from build123d import *

# Parameters (mm, degrees)
F1_DEPTH = 80
F2_R     = 2.25
F3_DEPTH = 3
F4_R     = 1.49999


# Not quite as in the source:
# - a fillet or chamfer is up to 0.001 mm smaller than in the source, because OpenCascade refuses the exact size
# - a feature names something its author has since deleted; it is built from what else it names


with BuildPart() as f1:
    # F0 (on Top) → F1 (new body)
    with BuildSketch(Plane.XY):
        with BuildLine():
            Line((45, 3), (3, 3))
            Line((3, 3), (3, 6))
            ThreePointArc((3, 6), (29.6273152762, 21.5830013932), (60, 27))
            Line((60, 27), (60, 30))
            ThreePointArc((60, 30), (27.9372056463, 24.1546059211), (0, 7.3705672421))
            Line((0, 7.3705672421), (0, 0))
            Line((0, 0), (45, 0))
            Line((45, 0), (45, 3))
        make_face()
    extrude(amount=F1_DEPTH)

    # F2 (on face) → F3 (cut, through all)
    with BuildSketch(Plane.XZ):
        with Locations((30, 72)):
            Circle(F2_R)
        with Locations((30, 8)):
            Circle(F2_R)
    extrude(amount=-F3_DEPTH, mode=Mode.SUBTRACT)

    # F4 (radius 1.5 in the source; OpenCascade refuses exactly that, so slightly less here)
    f4_edges = [f1.edges().sort_by_distance(p)[0] for p in [
        (45, 0, 40),
        (45, 3, 40),
        (0, 0, 40),
        (0, 7.370567, 40),
        (60, 30, 40),
        (60, 27, 40),
        (3, 3, 40),
        (3, 6, 40),
    ]]
    fillet(f4_edges, radius=F4_R)


solid = f1.part
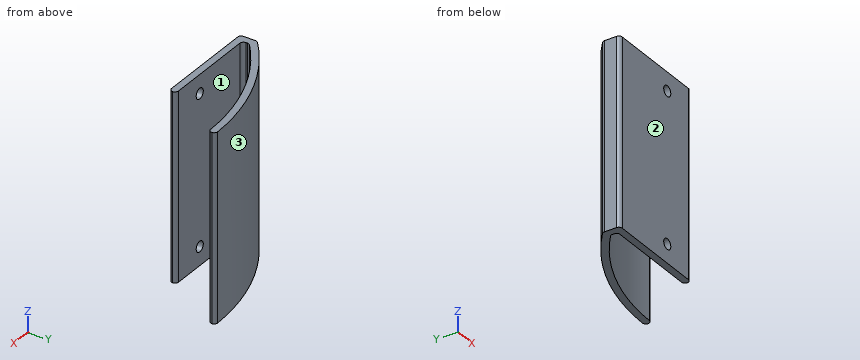
CAD build for the part. Positions are in the model's coordinates, mm. Face numbers are marked on the shaded views. Coordinates: 2 decimals unless noted, no trailing zeros. Loops run counter-clockwise (first coordinate to the right, second up) from the corner with the lowest first, then second, coordinate; pieces in that order, holes last. Notation, with made-up numbers: (77, 57.5) - (128, 57.5) arc R15 cw to (128, 66.5) - close; hole circle Ø1 at (18.5, 79). An arc over 180 degrees is marked (long way). Use one line per item in the form item = value. Start each with the question number.
1) Two-plate mould, pull along Y, no slides. Class the marked faces 1, 2 and 3: +Y half, -Y half, draft (parallel to the pull), parting line (faces both ways), or undercut.
2) Flat gauge pins, fed straight in: pin 1 (4 mm diameter, centred on x = 30, z = 72, fed in from -Y); pin 2 (5 mm diameter, centred on x = 50, z = 72, fed in from -Y); pin 3 (5 mm diameter, centred on y = 22.5, z = 59.5, fed in from -X). Where does each tip first touch, or does it go through?
3) Band-saw the part on D-D (x = 30). Give the cut face in (y, z), and give its area (3 significant figures).
4) Band-saw the part on B-B (x = 11.5). Give the cut face in (y, z).
5) Drill centre lines: L1, parallel to Z at x = 30, y = 0.9; L2, parallel to Y at x = 27.5, z = 75; L3, parallel to Y at x = 4.5, z = 47. Where is each one in solid material? Low to high. Write a range as from..to.
Check values:
q1.face_1 = undercut
q1.face_2 = -Y half
q1.face_3 = +Y half
q2.pin_1 = 20.97
q2.pin_2 = 26.11
q2.pin_3 = 18.56
q3.outline = (0, 0) - (3, 0) - (3, 5.75) - (0, 5.75) - close; (0, 10.25) - (3, 10.25) - (3, 69.75) - (0, 69.75) - close; (0, 74.25) - (3, 74.25) - (3, 80) - (0, 80) - close; (21.72, 0) - (24.9, 0) - (24.9, 80) - (21.72, 80) - close
q3.area = 468 mm2
q4.outline = (0, 0) - (3, 0) - (3, 80) - (0, 80) - close; (12.4, 0) - (15.97, 0) - (15.97, 80) - (12.4, 80) - close
q5.L1 = 0..5.75, 10.25..69.75, 74.25..80
q5.L2 = 0..3, 20.77..23.99
q5.L3 = 0..3, 7.25..11.08
